from build123d import *

# Parameters (mm, degrees)
SKETCH1_R           = 17.5
SKETCH1_R_2         = 2.5
BOSS_EXTRUDE1_DEPTH = 24
SKETCH1_3_R         = 21
SKETCH1_3_R_2       = 17.5
BOSS_EXTRUDE2_DEPTH = 17
SKETCH1_6_R         = 40
SKETCH1_6_R_2       = 21
BOSS_EXTRUDE4_DEPTH = 5
SKETCH1_7_R         = 42
SKETCH1_7_R_2       = 40
BOSS_EXTRUDE5_DEPTH = 16
SKETCH2_R           = 2.5
CUT_EXTRUDE1_DEPTH  = 6
CUT_EXTRUDE2_DEPTH  = 3
CUT_EXTRUDE3_DEPTH  = 20


with BuildPart() as part:
    # Sketch1 → Boss-Extrude1 (new body)
    with BuildSketch(Plane(origin=(0, 0, 0), x_dir=(1, 0, 0), z_dir=(0, 1, 0))):
        Circle(SKETCH1_R)
        with Locations((-9.959292144, 5.75)):
            Circle(SKETCH1_R_2, mode=Mode.SUBTRACT)
        with Locations((9.959292144, 5.75)):
            Circle(SKETCH1_R_2, mode=Mode.SUBTRACT)
        with Locations((0, -11.5)):
            Circle(SKETCH1_R_2, mode=Mode.SUBTRACT)
    extrude(amount=BOSS_EXTRUDE1_DEPTH)

    # Sketch1<3> → Boss-Extrude2 (add)
    with BuildSketch(Plane(origin=(0, 0, 0), x_dir=(1, 0, 0), z_dir=(0, 1, 0))):
        Circle(SKETCH1_3_R)
        Circle(SKETCH1_3_R_2, mode=Mode.SUBTRACT)
    extrude(amount=BOSS_EXTRUDE2_DEPTH)

    # Sketch1<6> → Boss-Extrude4 (add)
    with BuildSketch(Plane(origin=(0, 0, 0), x_dir=(1, 0, 0), z_dir=(0, 1, 0))):
        Circle(SKETCH1_6_R)
        Circle(SKETCH1_6_R_2, mode=Mode.SUBTRACT)
    extrude(amount=BOSS_EXTRUDE4_DEPTH)

    # Sketch1<7> → Boss-Extrude5 (add)
    with BuildSketch(Plane(origin=(0, 0, 0), x_dir=(1, 0, 0), z_dir=(0, 1, 0))):
        Circle(SKETCH1_7_R)
        Circle(SKETCH1_7_R_2, mode=Mode.SUBTRACT)
    extrude(amount=BOSS_EXTRUDE5_DEPTH)

    # Sketch2 → Cut-Extrude1 (cut, through all)
    with BuildSketch(Plane(origin=(0, 5, 0), x_dir=(1, 0, 0), z_dir=(0, 1, 0))):
        with Locations((-35, 0)):
            Circle(SKETCH2_R)
        with Locations((-17.5, 30.310889132)):
            Circle(SKETCH2_R)
        with Locations((17.5, 30.310889132)):
            Circle(SKETCH2_R)
        with Locations((35, 0)):
            Circle(SKETCH2_R)
        with Locations((17.5, -30.310889132)):
            Circle(SKETCH2_R)
        with Locations((-17.5, -30.310889132)):
            Circle(SKETCH2_R)
    extrude(amount=-CUT_EXTRUDE1_DEPTH, mode=Mode.SUBTRACT)

    # Sketch3 → Cut-Extrude2 (cut)
    with BuildSketch(Plane(origin=(0, 5, 0), x_dir=(1, 0, 0), z_dir=(0, 1, 0))):
        Polygon((-12.881197846, 30.310889132), (-15.190598923, 34.310889132), (-19.809401077, 34.310889132), (-22.118802154, 30.310889132), (-19.809401077, 26.310889132), (-15.190598923, 26.310889132), align=None)
        Polygon((19.809401077, 26.310889132), (22.118802154, 30.310889132), (19.809401077, 34.310889132), (15.190598923, 34.310889132), (12.881197846, 30.310889132), (15.190598923, 26.310889132), align=None)
        Polygon((32.690598923, -4), (37.309401077, -4), (39.618802154, 0), (37.309401077, 4), (32.690598923, 4), (30.381197846, 0), align=None)
        Polygon((12.881197846, -30.310889132), (15.190598923, -34.310889132), (19.809401077, -34.310889132), (22.118802154, -30.310889132), (19.809401077, -26.310889132), (15.190598923, -26.310889132), align=None)
        Polygon((-19.809401077, -26.310889132), (-22.118802154, -30.310889132), (-19.809401077, -34.310889132), (-15.190598923, -34.310889132), (-12.881197846, -30.310889132), (-15.190598923, -26.310889132), align=None)
        Polygon((-32.690598923, 4), (-37.309401077, 4), (-39.618802154, 0), (-37.309401077, -4), (-32.690598923, -4), (-30.381197846, 0), align=None)
    extrude(amount=-CUT_EXTRUDE2_DEPTH, mode=Mode.SUBTRACT)

    # Sketch4 → Cut-Extrude3 (cut)
    with BuildSketch(Plane.XZ):
        Polygon((0, 6.881197846), (4, 9.190598923), (4, 13.809401077), (0, 16.118802154), (-4, 13.809401077), (-4, 9.190598923), align=None)
        Polygon((5.959292144, -3.440598923), (5.959292144, -8.059401077), (9.959292144, -10.368802154), (13.959292144, -8.059401077), (13.959292144, -3.440598923), (9.959292144, -1.131197846), align=None)
        Polygon((-5.959292144, -3.440598923), (-9.959292144, -1.131197846), (-13.959292144, -3.440598923), (-13.959292144, -8.059401077), (-9.959292144, -10.368802154), (-5.959292144, -8.059401077), align=None)
    extrude(amount=-CUT_EXTRUDE3_DEPTH, mode=Mode.SUBTRACT)


solid = part.part
Here's how the part is built. I have some questions about the finished solid (model axes, mm). A direction names the side the tool comes from. Give positions to 0.01 mm unless a question says otherwise; leave off trailing zeros. Write each loop counter-clockwise with the first axis right and the second up, starting at its lowest first coordinate (ties: lowest second). Pieces come first, ordered by that corner, then holes. Notation, with made-up numbers: (65.25, 50.25) -> (99.25, 50.25) arc R9 ccw to (99.25, 59.25) -> close; hole circle Ø11 at (-22, 54). An arc over 180 degrees is marked (long way). Use one line per item in the form item = value. Start each with the question number.
1. Imagine slicing it at B-B on x = 35. List the corners of the cut face in (y, z) for me.
2. Will these pins go through, and if not, where does the flat tip stop? pin 1 Ø5 at (x, z) = (10, -19.5) entering from +Y; pin 2 Ø4 at (y, z) = (12, -23) entering from +X; pin 3 Ø3 at (x, z) = (9.96, -5.75) entering from -Y; pin 4 Ø3.5 at (x, y) = (-34.5, 3) entering from +Z.
3. On a 3-axis mill with a long thin cutter (end or side, diameter ignored), from which of +Z, -Z, +X, -X, +Y, -Y can I reach the whole of each face in a straight line? I mean faces 1 (the face through (-1.8, 20, 9.5)), 2 (the face through (38.48, 3.52, -1.97)), 3 (the face through (-18.04, 1.01, 32.75)). Say none if no direction works.
4. Imagine slicing it at C-C on x = -26. List the corners of the cut face in (y, z) for me, plus the area to 3 significant figures.
5. Imagine slicing it at A-A on y = 7.75. List the corners of the cut face in (x, z) for me, plus the area to 3 significant figures.
6. If I drill on L1, parallel to Z at x = 0, y = 22.25; L2, parallel to X at y = 9, z = 0; L3, parallel to X at y = 21.7, z = -5.75, over which ranges is the centre line in solid material (lowest first)?
7. Thinking about a two-plate mould opening in X: for faces 4 (the face through (2.028, 9.86, 14.948)), 5 (the face through (0, 24, 0)), which applies, +X half, -X half, draft (parallel to the pull), parting line (faces both ways), or undercut?
8. Imagine slicing it at D-D on y = 22.5. List the corners of the cut face in (x, z) for me, plus the area to 3 significant figures.
Entries:
q1.outline = (0, -23.22) -> (16, -23.22) -> (16, -19.36) -> (5, -19.36) -> (5, -4) -> (2, -4) -> (2, -2.5) -> (0, -2.5) -> close; (0, 2.5) -> (2, 2.5) -> (2, 4) -> (5, 4) -> (5, 19.36) -> (16, 19.36) -> (16, 23.22) -> (0, 23.22) -> close
q2.pin_1 = 17
q2.pin_2 = 36.37
q2.pin_3 = through
q2.pin_4 = 26.3
q3.face_1 = -Y
q3.face_2 = +Y
q3.face_3 = +Y, -Y
q4.outline = (0, -32.98) -> (16, -32.98) -> (16, -30.4) -> (5, -30.4) -> (5, 30.4) -> (16, 30.4) -> (16, 32.98) -> (0, 32.98) -> close
q4.area = 387 mm²
q5.outline = circle Ø84 at (0, 0); circle Ø42 at (0, 0); hole circle Ø80 at (0, 0); hole (-13.96, -8.06) -> (-9.96, -10.37) -> (-5.96, -8.06) -> (-5.96, -3.44) -> (-9.96, -1.13) -> (-13.96, -3.44) -> close; hole (-4, 9.19) -> (0, 6.88) -> (4, 9.19) -> (4, 13.81) -> (0, 16.12) -> (-4, 13.81) -> close; hole (5.96, -8.06) -> (9.96, -10.37) -> (13.96, -8.06) -> (13.96, -3.44) -> (9.96, -1.13) -> (5.96, -3.44) -> close
q5.area = 1,730 mm²
q6.L1 = -17.5 to 9, 14 to 17.5
q6.L2 = -42 to -40, -21 to 21, 40 to 42
q6.L3 = -16.53 to -12.46, -7.46 to 7.46, 12.46 to 16.53
q7.face_4 = undercut
q7.face_5 = draft
q8.outline = circle Ø35 at (0, 0); hole circle Ø5 at (-9.96, -5.75); hole circle Ø5 at (0, 11.5); hole circle Ø5 at (9.96, -5.75)
q8.area = 903 mm²
